Work out the finished part from the listing and answer in its coordinate system (mm). A direction names the side the tool comes from. Coordinates: 2 decimals unless noted, no trailing zeros. Write each loop counter-clockwise with the first axis right and the second up, starting at its lowest first coordinate (ties: lowest second). Pieces come first, ordered by that corner, then holes. Notation, with made-up numbers: M -3,80 L 53,80 A15 cw 53,85 Z; hole C 88,-10 d3. An arc over 180 degrees is marked long. Answer as CSV lines item,"result". Start each with the question number.
(1) Find the intervals of material crossed by L1, parallel to Y at x = -86.5, z = -33; L2, parallel to Z at x = 32, y = -63.5; L3, parallel to X at y = -40.5, z = -158.5, in increasing order. Write a range as [from, to].
(2) A cutting plane is placed at C-C on y = -78. Give the vertices of the cut face in (x, z).
(3) Flat-ended cylindrical pins translate along their axes: P1, Ø2.5, axis at y = -4, z = 58, coming from the -X side; P2, Ø10, axis at x = -86.5, z = -53, coming from the -Y side; P3, Ø9, axis at y = -4, z = -264, coming from the +X side. Find the tip coordinate at first contact, or state that the pin passes through.
(4) A cutting plane is placed at B-B on x = 50. Give the vertices of the cut face in (y, z), then the cut area to 3 significant figures.
(5) The mould has two halves that part along X. Classify faces 1 (the flat face through (-2, -12, -180)), 2 (the cylindrical face through (-50, -4, 150)), 3 (the flat face through (-83.13, -3.94, -332.69)), 4 (the cylindrical face through (20.08, -42.89, -141.6)): released by +X, released by -X, zero draft, split by the parting line, or undercut.
(6) For faces 5 (the flat face through (-76, -8, 5)), 6 (the flat face through (49.574, -93.752, -171.294)), 7 (the flat face through (47, -89, 200)), 8 (the cylindrical face through (-1.339, -2.085, 2.52)), 9 (the cylindrical face through (-50, -4, -150)), determine the directions among +Z, -Z, +X, -X, +Y, -Y from which every point of the face is accessible in a straight line to the end or side of a thin tool.
(7) A cutting plane is placed at D-D on z = -282. Give the vertices of the cut face in (x, y), then the cut area to 3 significant figures.
(8) A cutting plane is placed at A-A on z = -32. Give the vertices of the cut face in (x, y), then the cut area to 3 significant figures.
from build123d import *

# Parameters (mm, degrees)
SM_BASE_FLANGE_1_DEPTH = 350
CUT_EXTRUDE_1_DEPTH    = 10
CUT_EXTRUDE_2_DEPTH    = 10
CUT_EXTRUDE_START      = 180
CUT_EXTRUDE_3_DEPTH    = 170
CUT_EXTRUDE_4_DEPTH    = 10
SKETCH_10_W            = 150
SKETCH_10_H            = 123.452994616
CUT_EXTRUDE_5_DEPTH    = 10
SKETCH_11_W            = 20
SKETCH_11_H            = 53.452994616
CUT_EXTRUDE_6_DEPTH    = 10
CUT_EXTRUDE_7_DEPTH    = 10
FILLET_1_R             = 60
FILLET_2_R             = 30
FILLET_3_R             = 20


# Read off the part's stored shape, not the designer's step: 切除-拉伸3
# Sheet-metal steps are written as plain solids
with BuildPart() as part:
    # Sketch 1 → 基体-法兰1 (new, symmetric)
    with BuildSketch(Plane.XY):
        with BuildLine():
            Line((-120, 0), (-9.237604307, 0))
            ThreePointArc((-9.237604307, 0), (-1.237604307, -2.143593539), (4.618802154, -8))
            Line((4.618802154, -8), (67.5, -116.913429511))
            Line((67.5, -116.913429511), (60.57179677, -120.913429511))
            Line((60.57179677, -120.913429511), (-2.309401077, -12))
            ThreePointArc((-2.309401077, -12), (-5.237604307, -9.07179677), (-9.237604307, -8))
            Line((-9.237604307, -8), (-120, -8))
            Line((-120, -8), (-120, 0))
        make_face()
    extrude(amount=SM_BASE_FLANGE_1_DEPTH, both=True)

    # 草图6 → 切除-拉伸1 (cut)
    with BuildSketch(Plane(origin=(0, 0, 0), x_dir=(1, 0, 0), z_dir=(0, 1, 0))):
        Polygon((-120, -180), (-120, 180), (-100, 150), (-100, -150), align=None)
    extrude(amount=-CUT_EXTRUDE_1_DEPTH, mode=Mode.SUBTRACT)

    # 草图7 → 切除-拉伸2 (cut)
    with BuildSketch(Plane(origin=(0, 0, 0), x_dir=(1, 0, 0), z_dir=(0, 1, 0))):
        with BuildLine():
            Line((-65, -135), (-65, 135))
            ThreePointArc((-65, 135), (-50, 150), (-35, 135))
            Line((-35, 135), (-35, -135))
            ThreePointArc((-35, -135), (-50, -150), (-65, -135))
        make_face()
    extrude(amount=-CUT_EXTRUDE_2_DEPTH, mode=Mode.SUBTRACT)

    # 切除-拉伸3 outline → 切除-拉伸3 (cut)
    with BuildSketch(Plane.XY.offset(CUT_EXTRUDE_START)):
        with BuildLine():
            Line((-2.309401077, -12), (-1.154700538, -14))
            Line((-1.154700538, -14), (5.773502692, -10))
            Line((5.773502692, -10), (4.618802154, -8))
            ThreePointArc((4.618802154, -8), (-1.237604307, -2.143593539), (-9.237604307, 0))
            Line((-9.237604307, 0), (-55, 0))
            Line((-55, 0), (-55, -8))
            Line((-55, -8), (-9.237604307, -8))
            ThreePointArc((-9.237604307, -8), (-5.237604307, -9.07179677), (-2.309401077, -12))
        make_face()
    cut_extrude_3 = extrude(amount=CUT_EXTRUDE_3_DEPTH, mode=Mode.SUBTRACT)

    # 草图9 → 切除-拉伸4 (cut)
    with BuildSketch(Plane(origin=(0, 0, 0), x_dir=(1, 0, 0), z_dir=(0, 1, 0))):
        Polygon((-120, -350), (-120, -310), (-55, -350), align=None)
    cut_extrude_4 = extrude(amount=-CUT_EXTRUDE_4_DEPTH, mode=Mode.SUBTRACT)

    # 草图10 → 切除-拉伸5 (cut)
    with BuildSketch(Plane(origin=(0, 0, 0), x_dir=(0, 0, -1), z_dir=(0.8660254037844398, 0.49999999999999806, 0))):
        with Locations((-275, -73.273502692)):
            Rectangle(SKETCH_10_W, SKETCH_10_H)
    cut_extrude_5 = extrude(amount=-CUT_EXTRUDE_5_DEPTH, mode=Mode.SUBTRACT)

    # 草图11 → 切除-拉伸6 (cut)
    with BuildSketch(Plane(origin=(0, 0, 0), x_dir=(0, 0, -1), z_dir=(0.8660254037844398, 0.49999999999999806, 0))):
        with Locations((-190, -38.273502692)):
            Rectangle(SKETCH_11_W, SKETCH_11_H)
    cut_extrude_6 = extrude(amount=-CUT_EXTRUDE_6_DEPTH, mode=Mode.SUBTRACT)

    # 镜向1: 切除-拉伸4, 切除-拉伸5 across plane
    add(cut_extrude_4.mirror(Plane.XY), mode=Mode.SUBTRACT)
    add(cut_extrude_5.mirror(Plane.XY), mode=Mode.SUBTRACT)

    # 镜向2: 切除-拉伸3 across plane
    add(cut_extrude_3.mirror(Plane.XY), mode=Mode.SUBTRACT)

    # 镜向3: 切除-拉伸6 across plane
    add(cut_extrude_6.mirror(Plane.XY), mode=Mode.SUBTRACT)

    # 草图12 → 切除-拉伸7 (cut)
    with BuildSketch(Plane(origin=(0, 0, 0), x_dir=(0, 0, -1), z_dir=(0.8660254037844398, 0.49999999999999806, 0))):
        Polygon((-150, -35), (150, -35), (180, -135), (-180, -135), align=None)
    extrude(amount=-CUT_EXTRUDE_7_DEPTH, mode=Mode.SUBTRACT)

    # 圆角1
    fillet_1_edges = [part.edges().sort_by_distance(p)[0] for p in [
        (14.035898385, -32.310889132, 150),
        (14.035898385, -32.310889132, -150),
    ]]
    fillet(fillet_1_edges, radius=FILLET_1_R)

    # 圆角2
    fillet_2_edges = [part.edges().sort_by_distance(p)[0] for p in [
        (-120, -4, -180),
        (-100, -4, -150),
        (-100, -4, 150),
        (-120, -4, 180),
    ]]
    fillet(fillet_2_edges, radius=FILLET_2_R)

    # 圆角3
    fillet_3_edges = [part.edges().sort_by_distance(p)[0] for p in [
        (-120, -4, 310),
        (-120, -4, -310),
    ]]
    fillet(fillet_3_edges, radius=FILLET_3_R)


solid = part.part
Here are the results:
1,L1,"y = [-8, 0]"
1,L2,"z = [-200, -160.35], [160.35, 200]"
1,L3,"x = [14.15, 23.38]"
2,outline,"M 35.8,-200 L 45.03,-200 L 45.03,-166.52 L 35.8,-165.13 Z; M 35.8,165.13 L 45.03,166.52 L 45.03,200 L 35.8,200 Z"
3,P1,"stops at x = -100"
3,P2,"stops at y = -8"
3,P3,"stops at x = -55"
4,outline,"M -102.6,-200 L -86.6,-200 L -86.6,-169.5 L -102.6,-173.66 Z; M -102.6,173.66 L -86.6,169.5 L -86.6,200 L -102.6,200 Z"
4,area,"909 mm^2"
5,face 1,"zero draft"
5,face 2,"undercut"
5,face 3,"released by -X"
5,face 4,"released by +X"
6,face 5,"+Z, -Z, -X, -Y"
6,face 6,"+X, -Y"
6,face 7,"+Z, +X, -X, +Y, -Y"
6,face 8,"+Z, -Z, +X, +Y"
6,face 9,"+Y, -Y"
7,outline,"M -120,-8 L -55,-8 L -55,0 L -120,0 Z"
7,area,"520 mm^2"
8,outline,"M -100,-8 L -65,-8 L -65,0 L -100,0 Z; M -35,-8 L -9.24,-8 A8 cw -2.31,-12 L 10.57,-34.31 L 17.5,-30.31 L 4.62,-8 A16 ccw -9.24,0 L -35,0 Z"
8,area,"793 mm^2"
